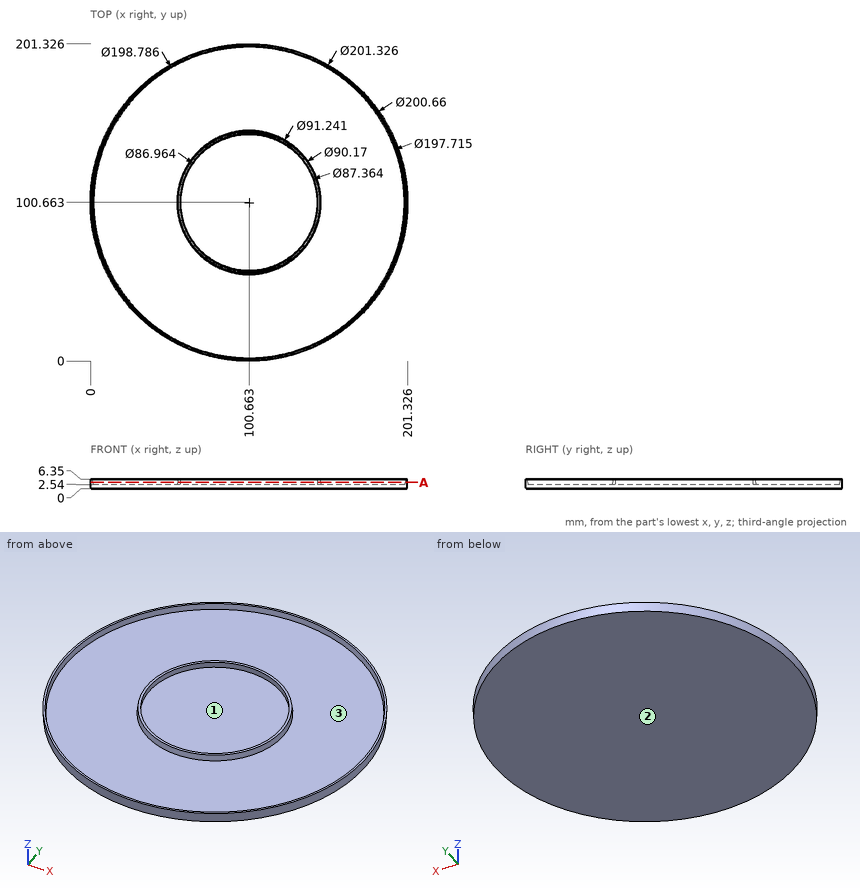
The figure shows three views and two pictorial views of one solid part (mm, origin at its lowest corner). Answer the questions. Coordinates: 2 decimals unless noted, no trailing zeros. Order: outer loops, then holes, each group sorted by start corner. A loop starts at its lowest first (then second) coordinate and runs counter-clockwise, first axis right, second up. Notation, with made-up numbers: (-40, 37) - (11, 37) arc R17 ccw to (11, 65) - close; hole circle Ø5 at (85, 75). An arc over 180 degrees is marked (long way). Answer as a JSON object with one key per item and string values.
1. Each of these flat-tipped pins is pushed along its axis until it touches: P1, Ø1, axis at x = 99.5, y = 112, coming from the +Z side; P2, Ø1, axis at x = 171.5, z = 2, coming from the -Y side; P3, Ø1, axis at y = 71.5, z = 1.5, coming from the +X side. Where does it stop, or does it pass through?
Output values:
{"P1": "stops at z = 2.54", "P2": "stops at y = 28.97", "P3": "stops at x = 196.9"}
2. Find section A-A on z = 4.25. Determine the outline of the cut face in (x, y) (1 decimal).
Output values:
{"outline": "circle Ø201.1 at (100.7, 100.7); circle Ø90.8 at (100.7, 100.7); hole circle Ø198.2 at (100.7, 100.7); hole circle Ø87.2 at (100.7, 100.7)"}
3. Consider line 1 (Y direction, x = 113, z = 5.75) (1 decimal); line 2 (Y direction, x = 139.5, z = 5.5) (1 decimal); line 3 (X direction, y = 96, z = 5.75) (1 decimal). Determine where each line is inside the solid, lowest interval first.
Output values:
{"line 1": "y = 0.8 to 2.1, 57.2 to 58.9, 142.4 to 144.1, 199.2 to 200.5", "line 2": "y = 7.8 to 9.3, 77.5 to 81, 120.3 to 123.8, 192 to 193.5", "line 3": "x = 0.1 to 1.5, 55.7 to 57.4, 143.9 to 145.6, 199.9 to 201.2"}
4. The mould has two halves that part along Y. Classify the marked faces 1, 2 and 3: +Y half, -Y half, draft (parallel to the pull), parting line (faces both ways), or undercut.
Output values:
{"face 1": "undercut", "face 2": "draft", "face 3": "undercut"}
